```python
from build123d import *

# Parameters (mm, degrees)
F0_W     = 24
F0_H     = 12
F0_W_2   = 19.8
F0_H_2   = 9.4
F1_DEPTH = 0.9
F2_W     = 24
F2_H     = 12
F3_DEPTH = 2.7
F4_R     = 1.6
F5_DEPTH = 1.2
F6_R     = 0.2
F7_R     = 0.8
F8_DEPTH = 5


with BuildPart() as f1:
    # F0 (on Top) → F1 (new body)
    with BuildSketch(Plane.XY):
        Rectangle(F0_W, F0_H)
        Rectangle(F0_W_2, F0_H_2, mode=Mode.SUBTRACT)
    extrude(amount=F1_DEPTH)

    # F2 (on face) → F3 (join)
    with BuildSketch(Plane(origin=(0, 0, 0), x_dir=(1, 0, 0), z_dir=(0, 0, -1))):
        Rectangle(F2_W, F2_H)
    extrude(amount=F3_DEPTH)

    # F4 (on face) → F5 (cut)
    with BuildSketch(Plane(origin=(0, 0, -2.7), x_dir=(1, 0, 0), z_dir=(0, 0, -1))):
        Circle(F4_R)
        with Locations((-9, 0)):
            Circle(F4_R)
        with Locations((9, 0)):
            Circle(F4_R)
    extrude(amount=-F5_DEPTH, mode=Mode.SUBTRACT)

    # F6
    f6_edges = [f1.edges().sort_by_distance(p)[0] for p in [
        (-12, -6, -0.9),
        (-12, 6, -0.9),
        (12, 6, -0.9),
        (12, -6, -0.9),
    ]]
    fillet(f6_edges, radius=F6_R)

    # F7 (on face) → F8 (cut)
    with BuildSketch(Plane.XZ.offset(6)):
        with Locations((-6.5, -1.3)):
            Circle(F7_R)
        with Locations((6.5, -1.3)):
            Circle(F7_R)
    extrude(amount=-F8_DEPTH, mode=Mode.SUBTRACT)


solid = f1.part
```
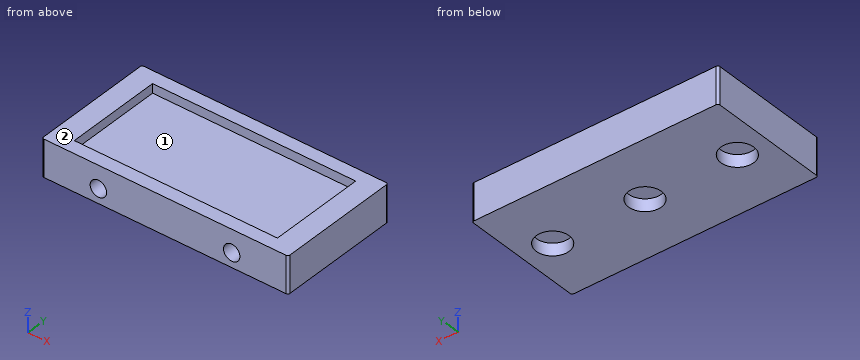
Can you work these out from the model? Positions are in its coordinate system, mm. Face numbers are marked on the shaded views. A direction names the side the tool comes from. Give positions to 0.01 mm unless a question says otherwise; leave off trailing zeros. Loops run counter-clockwise (first coordinate to the right, second up) from the corner with the lowest first, then second, coordinate; pieces in that order, holes last. Notation, with made-up numbers: M 82.25,22.5 L 102.25,22.5 A33 ccw 102.25,52.5 Z; hole C 8,-17.75 d11. An arc over 180 degrees is marked long. Use one line per item in the form item = value. Start each with the question number.
(1) I want a section at B-B, the plane z = -2.45. Write out the boundary of the cut face in (x, y), and give its area (3 significant figures).
(2) I want a section at C-C, the plane y = 3. Write out the boundary of the cut face in (x, z), and give its area (3 significant figures).
(3) Please list where these lines run through material, in increasing order: line 1 (X direction, y = 0, z = -1.75); line 2 (X direction, y = -4, z = 0.6); line 3 (X direction, y = -4.25, z = -1.5).
(4) I'm going to push flat-ended pins straight in: P1, Ø3, axis at x = 0, y = 0, coming from the -Z side; P2, Ø1.3, axis at x = 6.5, z = -1.3, coming from the -Y side; P3, Ø1, axis at x = -5, y = -3, coming from the +Z side. Where does each tip first touch, or does it pass through?
(5) On a 3-axis mill with a long thin cutter (end or side, diameter ignored), from which of +Z, -Z, +X, -X, +Y, -Y can I reach the whole of each face in a straight line? I mean the marked faces 1 and 2. Say none if no direction works.
(6) I want a section at A-A, the plane x = 2.5. Write out the boundary of the cut face in (y, z).
(7) I want a section at D-D, the plane y = -5. Write out the boundary of the cut face in (x, z).
Worked out:
q1.outline = M -12,-5.8 A0.2 ccw -11.8,-6 L 11.8,-6 A0.2 ccw 12,-5.8 L 12,5.8 A0.2 ccw 11.8,6 L -11.8,6 A0.2 ccw -12,5.8 Z; hole C -9,0 d3.2; hole C 0,0 d3.2; hole C 9,0 d3.2
q1.area = 264 mm²
q2.outline = M -12,-2.7 L 12,-2.7 L 12,0.9 L 9.9,0.9 L 9.9,0 L -9.9,0 L -9.9,0.9 L -12,0.9 Z
q2.area = 68.6 mm²
q3.line_1 = -12 to -10.6, -7.4 to -1.6, 1.6 to 7.4, 10.6 to 12
q3.line_2 = -12 to -9.9, 9.9 to 12
q3.line_3 = -12 to -7.27, -5.73 to 5.73, 7.27 to 12
q4.P1 = -1.5
q4.P2 = -1
q4.P3 = 0
q5.face_1 = +Z
q5.face_2 = +Z, +X, -X, +Y, -Y
q6.outline = M -6,-2.7 L 6,-2.7 L 6,0.9 L 4.7,0.9 L 4.7,0 L -4.7,0 L -4.7,0.9 L -6,0.9 Z
q7.outline = M -12,-2.7 L 12,-2.7 L 12,0.9 L -12,0.9 Z; hole C -6.5,-1.3 d1.6; hole C 6.5,-1.3 d1.6
